from build123d import *

# Parameters (mm, degrees)
BOSS_EXTRUDE1_DEPTH = 20
CHAMFER1_START      = -5
CHAMFER1_OUTLINE_W  = 22
CHAMFER1_OUTLINE_H  = 11
CHAMFER1_DEPTH      = 1.687562561


with BuildPart() as part:
    # Sketch1 → Boss-Extrude1 (new body)
    with BuildSketch(Plane(origin=(0, 0, 0), x_dir=(1, 0, 0), z_dir=(0, 1, 0))):
        Polygon((0, 0), (4, 0), (4, 13), (7.3, 13), (7.3, 0), (11.3, 0), (11.3, 13), (0, 16.176286751), align=None)
    boss_extrude1 = extrude(amount=BOSS_EXTRUDE1_DEPTH)

    # Mirror1: Boss-Extrude1 across plane
    add(boss_extrude1.mirror(Plane(origin=(11.3, 20, -13), x_dir=(0.9626917464264807, 0, 0.2706004459758567), z_dir=(-0.2706004459758567, 0, 0.9626917464264807))))

    # Chamfer1: read off the stored shape, not the designer's step
    # Chamfer1 outline → Chamfer1 (cut)
    with BuildSketch(Plane(origin=(0, 0, 0), x_dir=(0, 1, 0), z_dir=(0.9626917464264807, 0, 0.2706004459758569)).offset(CHAMFER1_START)):
        with Locations((10, -15.5)):
            Rectangle(CHAMFER1_OUTLINE_W, CHAMFER1_OUTLINE_H)
    extrude(amount=CHAMFER1_DEPTH, mode=Mode.SUBTRACT)


solid = part.part
Here's how the part is built. I have some questions about the finished solid (model axes, mm). A direction names the side the tool comes from. Give positions to 0.01 mm unless a question says otherwise; leave off trailing zeros. Loops run counter-clockwise (first coordinate to the right, second up) from the corner with the lowest first, then second, coordinate; pieces in that order, holes last. Notation, with made-up numbers: (87, 69.25) -> (143, 69.25) arc R19 ccw to (143, 85.25) -> close; hole circle Ø4 at (79, 13). An arc over 180 degrees is marked (long way). Answer as a JSON object with one key per item and string values. Group by question number.
Item 1: Thinking about a two-plate mould opening in Z: for faces 1 (the flat face through (8.503, 9.86, -22.429)), 2 (the flat face through (16.342, 9.86, -25.153)), 3 (the flat face through (6, 10, -13)), which applies, pulls with the +Z half, pulls with the -Z half, needs draft (parallel to the pull), parting line crosses it, or undercut?
Item 2: Imagine slicing it at C-C on z = -25.5. Write out the boundary of the cut face in (x, y), then the cut area to 3 significant figures.
Item 3: Will these pins go through, and if not, where does the flat tip stop? pin 1 (4 mm diameter, centred on y = 14.5, z = -7.5, fed in from +X); pin 2 (10.5 mm diameter, centred on y = 13.5, z = -9, fed in from +X); pin 3 (8 mm diameter, centred on y = 5.5, z = -13.5, fed in from +X).
Item 4: Imagine slicing it at D-D on x = 4.5. Write out the boundary of the cut face in (y, z).
Item 5: Imagine slicing it at A-A on z = -7. Write out the boundary of the cut face in (x, y), then the cut area to 3 significant figures.
Item 6: I need wall thicknesses on L1, parallel to X at y = 18.25, z = -2; L2, parallel to Z at x = 9.5, y = 15; L3, parallel to X at y = 10, z = -24.25. Which ranges of each line are inside material? Lowest first, please.
Item 7: Imagine slicing it at B-B on y = 3.5. Write out the boundary of the cut face in (x, z), then the cut area to 3 significant figures.
Item 8: On a 3-axis mill with a long thin cutter (end or side, diameter ignored), from which of +Z, -Z, +X, -X, +Y, -Y can I reach the whole of each face in a straight line? I mean faces 4 (the flat face through (11.22, 9.86, -20.55)), 5 (the flat face through (11.3, 10, -6)), 6 (the flat face through (4, 10, -6)). Say none if no direction works.
Answer list:
{
 "1": {"face 1": "undercut", "face 2": "pulls with the -Z half", "face 3": "pulls with the +Z half"},
 "2": {"outline": "(5.69, 0) -> (10.38, 0) -> (10.38, 20) -> (5.69, 20) -> close; (14.24, 0) -> (15.77, 0) -> (15.77, 20) -> (14.24, 20) -> close", "area": "124 mm2"},
 "3": {"pin 1": "stops at x = 11.3", "pin 2": "stops at x = 12.06", "pin 3": "stops at x = 14.05"},
 "4": {"outline": "(0, -23.55) -> (20, -23.55) -> (20, -13) -> (0, -13) -> close"},
 "5": {"outline": "(0, 0) -> (4, 0) -> (4, 20) -> (0, 20) -> close; (7.3, 0) -> (11.3, 0) -> (11.3, 20) -> (7.3, 20) -> close", "area": "160 mm2"},
 "6": {"L1": "x = 0 to 4, 7.3 to 11.3", "L2": "z = -29.33 to -24.06, -17.73 to 0", "L3": "x = 4.93 to 9.61, 13.48 to 17.82"},
 "7": {"outline": "(0, -12.24) -> (2.05, -19.54) -> (8.43, -29.98) -> (11.84, -27.9) -> (5.07, -16.8) -> (7.89, -15.08) -> (14.66, -26.18) -> (18.07, -24.1) -> (11.3, -13) -> (11.3, 0) -> (7.3, 0) -> (7.3, -13) -> (4, -13) -> (4, 0) -> (0, 0) -> close", "area": "240 mm2"},
 "8": {"face 4": "+Y, -Y", "face 5": "+Z, +X, +Y, -Y", "face 6": "+Z, +Y, -Y"}
}
